Design review of the part built by this model. Coordinates are the model's own, in mm. A direction names the side the tool comes from. Coordinates: 2 decimals unless noted, no trailing zeros. Write each loop counter-clockwise with the first axis right and the second up, starting at its lowest first coordinate (ties: lowest second). Pieces come first, ordered by that corner, then holes. Notation, with made-up numbers: (23.5, 10.25) -> (31.5, 10.25) arc R19 ccw to (31.5, 33.25) -> close; hole circle Ø11 at (31.25, 61.5). An arc over 180 degrees is marked (long way). Answer in a Markdown table with one row per item. Add a question column.
Item 1: For faces 1 (the face through (6, 3.3, 0.1)), 2 (the face through (36, 0, 0)), 3 (the face through (2.465, -1.233, 2.175)), list the 3-axis set-ups (+Z, -Z, +X, -X, +Y, -Y) from which the entire face can be reached by the end or side of a thin tool; tool diameter is ignored.
Item 2: Draft analysis for pull direction Y (two halves, no side actions). For faces 4 (the face through (2.465, 1.233, -2.175)), 5 (the face through (0, 2, 2)), 6 (the face through (3.41, -1.08, -4.88)), state which applies: released by +Y, released by -Y, zero draft, split by the parting line, or undercut.
Item 3: Clearance check with flat-ended pins moving along their axes: P1, Ø1.5, axis at x = 19, y = 0, coming from the +Z side; P2, Ø2.5, axis at y = -0.5, z = 0.5, coming from the -X side; P3, Ø6, axis at x = 8.5, y = -2, coming from the +Z side. State where each tip first meets the part, or that it passes through.
Item 4: Take a section at A-A, the plane x = 3. Write out the cut boundary in (y, z), and give its area (3 significant figures).
Item 5: To check wall thickness, follow line 1 (X direction, y = -0.5, z = 1); line 2 (X direction, y = -1.5, z = -3.5); line 3 (Y direction, x = 3, z = -2). State the ranges of each line that lie inside material, in increasing order.
Item 6: Take a section at B-B, the plane z = 0. Write out the cut boundary in (x, y), and give its area (3 significant figures).
Autodesk Inventor part; units mm, degrees
ref_plane "YZ Plane" through (0, 0, 0) normal (1, 0, 0) x (0, 1, 0)
ref_plane "XZ Plane" through (0, 0, 0) normal (0, 1, 0) x (-1, 0, 0)
ref_plane "XY Plane" through (0, 0, 0) normal (0, 0, 1) x (1, 0, 0)
sketch "Sketch1" plane through (0, 0, 0) normal (0, 0, 1) x (1, 0, 0)
  line L0 (0, 6) -> (0, -1)
  line L1 (-7.2, 0) -> (43.2, 0)
  line L2 (0, 5) -> (6, 5)
  line L3 (6, 5) -> (6, 3)
  line L4 (6, 3) -> (36, 3)
  line L5 (36, 3) -> (36, 0)
  line L6 (0, 0) -> (36, 0)
  line L7 (0, 5) -> (0, 0)
  dimension "d0" = 30
  dimension "d1" = 10
  dimension "d2" = 6
  dimension "d3" = 6
revolve "Revolution1" add sketch "Sketch1" angle 360 about axis through (0, 0, 0) along (1, 0, 0)
sketch "Sketch2" plane through (0, 0, 0) normal (-1, 0, 0) x (0, 0, 1)
  line L0 (-7, 0) -> (7, 0)
  line L1 (0, 7) -> (0, -7)
  line L2 (1.4434, -2.5) -> (-1.4434, -2.5)
  line L3 (-1.4434, -2.5) -> (-2.8868, 0)
  line L4 (-2.8868, 0) -> (-1.4434, 2.5)
  line L5 (-1.4434, 2.5) -> (1.4434, 2.5)
  line L6 (1.4434, 2.5) -> (2.8868, 0)
  line L7 (2.8868, 0) -> (1.4434, -2.5)
  point P0 (0, 0)
  point P1 (0, 0)
  dimension "d5" = 5
extrude "Extrusion1" cut sketch "Sketch2" against normal blind 5
thread "Thread1"
chamfer "Chamfer1" distance 0.75 angle 45 2 edges at (0, -5, 0) (36, -3, 0)
properties part number "M6x30" material "Stainless Steel"
Answers:
| question | item | result |
|---|---|---|
| 1 | face 1 | +X |
| 1 | face 2 | +Z, -Z, +X, +Y, -Y |
| 1 | face 3 | -X |
| 2 | face 4 | undercut |
| 2 | face 5 | zero draft |
| 2 | face 6 | split by the parting line |
| 3 | P1 | stops at z = 3 |
| 3 | P2 | stops at x = 5 |
| 3 | P3 | stops at z = 4.99 |
| 4 | outline | circle Ø10 at (0, 0); hole (-2.5, -1.44) -> (0, -2.89) -> (2.5, -1.44) -> (2.5, 1.44) -> (0, 2.89) -> (-2.5, 1.44) -> close |
| 4 | area | 56.9 mm^2 |
| 5 | line 1 | x = 5 to 36 |
| 5 | line 2 | x = 0 to 6 |
| 5 | line 3 | y = -4.58 to -1.54, 1.54 to 4.58 |
| 6 | outline | (0, -4.25) -> (0.75, -5) -> (6, -5) -> (6, -3) -> (35.25, -3) -> (36, -2.25) -> (36, 2.25) -> (35.25, 3) -> (6, 3) -> (6, 5) -> (0.75, 5) -> (0, 4.25) -> (0, 2.5) -> (5, 2.5) -> (5, -2.5) -> (0, -2.5) -> close |
| 6 | area | 214 mm^2 |
